Autodesk Inventor part; units mm, degrees
ref_plane "YZ Plane" through (0, 0, 0) normal (1, 0, 0) x (0, 1, 0)
ref_plane "XZ Plane" through (0, 0, 0) normal (0, 1, 0) x (-1, 0, 0)
ref_plane "XY Plane" through (0, 0, 0) normal (0, 0, 1) x (1, 0, 0)
sketch "Sketch1" plane through (0, 0, 0) normal (0, 1, 0) x (-1, 0, 0)
  line L0 (3, 3) -> (-3, 3) construction
  line L1 (-3, 3) -> (-3, -3) construction
  line L2 (-3, -3) -> (3, -3) construction
  line L3 (3, -3) -> (3, 3) construction
  circle A0 centre (0, 0) radius 4.2426
  dimension "d2" = 6
  dimension "d3" = 6
  dimension "d4" = 3
  dimension "d5" = 3
extrude "Extrusion1" add sketch "Sketch1" along normal blind 15
sketch "Sketch2" plane through (0, 15, 0) normal (0, 1, 0) x (1, 0, 0)
  line L0 (-3, -3) -> (3, -3)
  line L1 (3, -3) -> (3, 3)
  line L2 (3, 3) -> (-3, 3)
  line L3 (-3, 3) -> (-3, -3)
  circle A0 centre (0, 0) radius 4.2426
  dimension "d8" = 6
  dimension "d9" = 6
  dimension "d22" = 3
extrude "Extrusion2" add sketch "Sketch2" along normal blind 4 contours L3 L2 L1 L0
chamfer "Chamfer1" distance 1 angle 60 1 edges at (4.2426, 0, 0) measured on face at (-1.1052, 0, 1.3223)
sketch "Sketch4" plane through (0, 19, 0) normal (0, 1, 0) x (1, 0, 0)
  point P0 (0, 0)
  point P1 (0, 0)
hole "Hole2" at (0, 19, 0) direction (0, -1, 0) diameter 2.6416 depth 7.01 tip angle 118
properties part number "motor_shaft"
Geometry check sheet. Reference: the model listing, model coordinates, mm. A direction names the side the tool comes from. Round coordinates to 2 decimals unless told otherwise and drop trailing zeros. Loops run counter-clockwise (first coordinate to the right, second up) from the corner with the lowest first, then second, coordinate; pieces in that order, holes last. Notation, with made-up numbers: (-39, 55) - (-34, 55) arc R12 cw to (-34, 73) - close; hole circle Ø9 at (88, -38). An arc over 180 degrees is marked (long way). Write each question's results on one line, items separated by ' | '. Start each with the question number.
Q1. Access from +Z, -Z, +X, -X, +Y, -Y to the whole of each face (thin tool, end or side, straight path). Record for faces 4 (the flat face through (-3, 17, 0)), 5 (the flat face through (3.5, 15, 0)), 6 (the flat face through (0, 15, 3.5)), 7 (the flat face through (0, 15, -3.5)).
Q2. Release check for a two-part mould opening along Z. For faces 1 (the cylindrical face through (3, 8, 3)), 2 (the conical face through (0.069, 11.334, 0.219)), 3 (the flat face through (0, 17, -3)) record: +Z half, -Z half, draft (parallel to the pull), parting line (faces both ways), or undercut.
Q3. Cross-section at A-A on y = 14. Enter the section's corners in (x, z), and give its area (3 significant figures).
Q4. Thickness scan on line 1 (Z direction, x = 0, y = 14.75); line 2 (Z direction, x = 0, y = 16.75). Record the ranges inside material, lowest first. Write a range as [from, to].
Q5. Cross-section at B-B on y = 2. Enter the section's corners in (x, z), and give its area (3 significant figures).
Q6. Gauge pin test, flat ends, axial feed: P1, Ø1.2, axis at x = -0.5, y = 16, coming from the -Z side; P2, Ø1.2, axis at y = 17.5, z = 0.5, coming from the +X side; P3, Ø1.2, axis at y = 17.5, z = 1.5, coming from the -X side. Record the tip position at first contact, or that the pin passes through.
Answers below:
1) face 4: +Z, -Z, -X, +Y | face 5: +Z, -Z, +X, +Y | face 6: +Z, +X, -X, +Y | face 7: -Z, +X, -X, +Y
2) face 1: parting line | face 2: undercut | face 3: -Z half
3) outline: circle Ø8.49 at (0, 0); hole circle Ø2.64 at (0, 0) | area: 51.1 mm²
4) line 1: z = [-4.24, -1.32], [1.32, 4.24] | line 2: z = [-3, -1.32], [1.32, 3]
5) outline: circle Ø8.49 at (0, 0) | area: 56.5 mm²
6) P1: stops at z = -3 | P2: stops at x = 3 | P3: stops at x = -3
